Work out the finished part from the listing and answer in its coordinate system (mm). Face numbers are marked on the shaded views. A direction names the side the tool comes from. Coordinates: 2 decimals unless noted, no trailing zeros. Write each loop counter-clockwise with the first axis right and the second up, starting at its lowest first coordinate (ties: lowest second). Pieces come first, ordered by that corner, then holes. Notation, with made-up numbers: (35, -32.75) - (39, -32.75) arc R25 ccw to (39, -17.75) - close; hole circle Ø6 at (75, -10.75). An arc over 180 degrees is marked (long way). Use one line per item in the form item = value. Start each with the question number.
Item 1: For the marked faces 4 and 5, determine the directions among +Z, -Z, +X, -X, +Y, -Y from which every point of the face is accessible in a straight line to the end or side of a thin tool.
Item 2: A cutting plane is placed at A-A (y = 0). Write down the section's boundary in (x, z).
Item 3: A cutting plane is placed at C-C (y = 18). Write down the section's boundary in (x, z), then the cut area to 3 significant figures.
Item 4: A cutting plane is placed at D-D (y = -6). Write down the section's boundary in (x, z), then the cut area to 3 significant figures.
Item 5: Consider probe 1 along Y at (x, z) = (0, -6.75); probe 2 along X at (y, z) = (17.5, -9.5); probe 3 along Y at (x, z) = (15, -14). Determine where each line is inside the solid, lowest interval first.
Item 6: Determine the mould class of the marked faces 1, 2 and 3 for opening direction Y: released by +Y, released by -Y, zero draft, split by the parting line, or undercut.
Item 7: Given pin 1 (4.5 mm diameter, centred on x = 17, z = -5.5, fed in from +Y); pin 2 (5 mm diameter, centred on x = 3.5, z = -6.5, fed in from -Y); pin 3 (4 mm diameter, centred on y = 17, z = -2, fed in from -X); pin 4 (1.8 mm diameter, centred on x = -24.18, y = 0, fed in from +Z) (3 decimals), each flat-ended and moving along its own axis, determine where each tip first touches the part or whether it passes through.
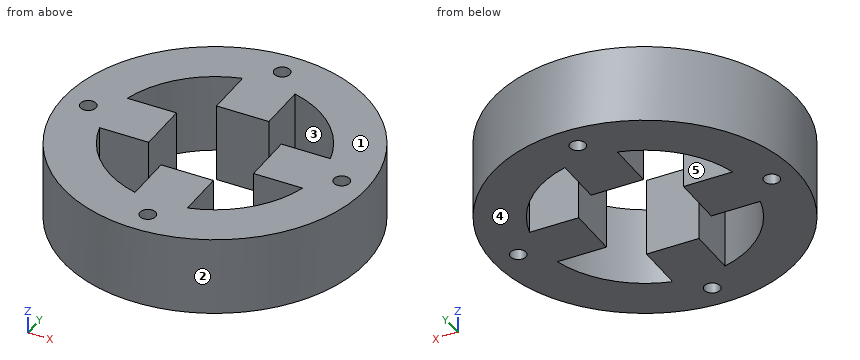
from build123d import *

# Parameters (mm, degrees)
SKETCH6_R                 = 29
SKETCH6_R_2               = 20
INNER_RING_DEPTH          = 15
MOTOR_CONNECTOR_CUT_DEPTH = 15
SKETCH8_R                 = 1.5
M3_HOLES_DEPTH            = 38
M3_HOLES_DEPTH_BACK       = 53


with BuildPart() as part:
    # Sketch6 → Inner Ring (new body)
    with BuildSketch(Plane.XY):
        Circle(SKETCH6_R)
        Circle(SKETCH6_R_2, mode=Mode.SUBTRACT)
    extrude(amount=-INNER_RING_DEPTH)

    # Sketch7 → Motor Connector Cut (add)
    with BuildSketch(Plane.XY):
        with BuildLine():
            ThreePointArc((20, 0), (19.840593925, 2.52008585), (19.364916731, 5))
            Line((19.364916731, 5), (9.999996731, 5))
            Line((9.999996731, 5), (9.999996731, -5))
            Line((9.999996731, -5), (19.364916731, -5))
            ThreePointArc((19.364916731, -5), (19.840593925, -2.52008585), (20, 0))
        make_face()
        with BuildLine():
            ThreePointArc((5, 19.364916731), (0, 20), (-5, 19.364916731))
            Line((-5, 19.364916731), (-5, 9.999996731))
            Line((-5, 9.999996731), (5, 9.999996731))
            Line((5, 9.999996731), (5, 19.364916731))
        make_face()
        with BuildLine():
            Line((-9.999996731, -5), (-9.999996731, 5))
            Line((-9.999996731, 5), (-19.364916731, 5))
            ThreePointArc((-19.364916731, 5), (-20, 0), (-19.364916731, -5))
            Line((-19.364916731, -5), (-9.999996731, -5))
        make_face()
        with BuildLine():
            Line((-5, -9.999996731), (-5, -19.364916731))
            ThreePointArc((-5, -19.364916731), (0, -20), (5, -19.364916731))
            Line((5, -19.364916731), (5, -9.999996731))
            Line((5, -9.999996731), (-5, -9.999996731))
        make_face()
    extrude(amount=-MOTOR_CONNECTOR_CUT_DEPTH)

    # Sketch8 → M3 Holes (cut, two sides)
    with BuildSketch(Plane.XY) as m3_holes_sk:
        with Locations((0, 24.182458366)):
            Circle(SKETCH8_R)
        with Locations((24.182458366, 0)):
            Circle(SKETCH8_R)
        with Locations((0, -24.182458366)):
            Circle(SKETCH8_R)
        with Locations((-24.182458366, 0)):
            Circle(SKETCH8_R)
    extrude(amount=M3_HOLES_DEPTH, mode=Mode.SUBTRACT)
    extrude(m3_holes_sk.sketch, amount=-M3_HOLES_DEPTH_BACK, mode=Mode.SUBTRACT)


solid = part.part
Answer:
q1.face_4 = -Z, +X, -X, +Y, -Y
q1.face_5 = +Z, -Z
q2.outline = (-29, -15) - (-25.68, -15) - (-25.68, 0) - (-29, 0) - close; (-22.68, -15) - (-10, -15) - (-10, 0) - (-22.68, 0) - close; (10, -15) - (22.68, -15) - (22.68, 0) - (10, 0) - close; (25.68, -15) - (29, -15) - (29, 0) - (25.68, 0) - close
q3.outline = (-22.74, -15) - (-8.72, -15) - (-8.72, 0) - (-22.74, 0) - close; (-5, -15) - (5, -15) - (5, 0) - (-5, 0) - close; (8.72, -15) - (22.74, -15) - (22.74, 0) - (8.72, 0) - close
q3.area = 571 mm²
q4.outline = (-28.37, -15) - (-19.08, -15) - (-19.08, 0) - (-28.37, 0) - close; (19.08, -15) - (28.37, -15) - (28.37, 0) - (19.08, 0) - close
q4.area = 279 mm²
q5.probe_1 = -29 to -25.68, -22.68 to -10, 10 to 22.68, 25.68 to 29
q5.probe_2 = -23.12 to -9.68, -5 to 5, 9.68 to 23.12
q5.probe_3 = -24.82 to -13.23, -5 to 5, 13.23 to 24.82
q6.face_1 = zero draft
q6.face_2 = split by the parting line
q6.face_3 = undercut
q7.pin_1 = 24.97
q7.pin_2 = -28.98
q7.pin_3 = -24.82
q7.pin_4 = through
